Geometry check sheet. Reference: drawing and pictorial views, mm from the part's lowest x, y, z. Round coordinates to 2 decimals unless told otherwise and drop trailing zeros. Order: outer loops, then holes, each group sorted by start corner. A loop starts at its lowest first (then second) coordinate and runs counter-clockwise, first axis right, second up.
(1) Release check for a two-part mould opening along X. For the marked faces 1, 2 and 3 record: +X half, -X half, draft (parallel to the pull), parting line (faces both ways), or undercut.
(2) Sectioned sample at D-D (x = 32.5). Record the boundary of the cut face in (y, z).
(3) Sectioned sample at C-C (z = 5). Record the boundary of the cut face in (x, y).
(4) Go/stop test with flat-tipped pins: pin 1 (2 mm diameter, centred on x = 28, y = 19.5, fed in from -Z); pin 2 (2 mm diameter, centred on x = 19.5, y = 27, fed in from +Z); pin 3 (0.7 mm diameter, centred on x = 12.5, z = 2.5, fed in from +Y); pin 4 (1.1 mm diameter, centred on y = 15, z = 2.5, fed in from -X). Record where each tip stops, or that it passes through.
(5) Sectioned sample at B-B (y = 33). Record the boundary of the cut face in (x, z).
(6) Material ranges on line 1 along X through (y, z) = (35, 2.75); line 2 along Y through (x, z) = (12.5, 1.75); line 3 along X through (y, z) = (24.5, 9), recorded low to high.
(7) Sectioned sample at A-A (x = 6.5). Record the boundary of the cut face in (y, z).
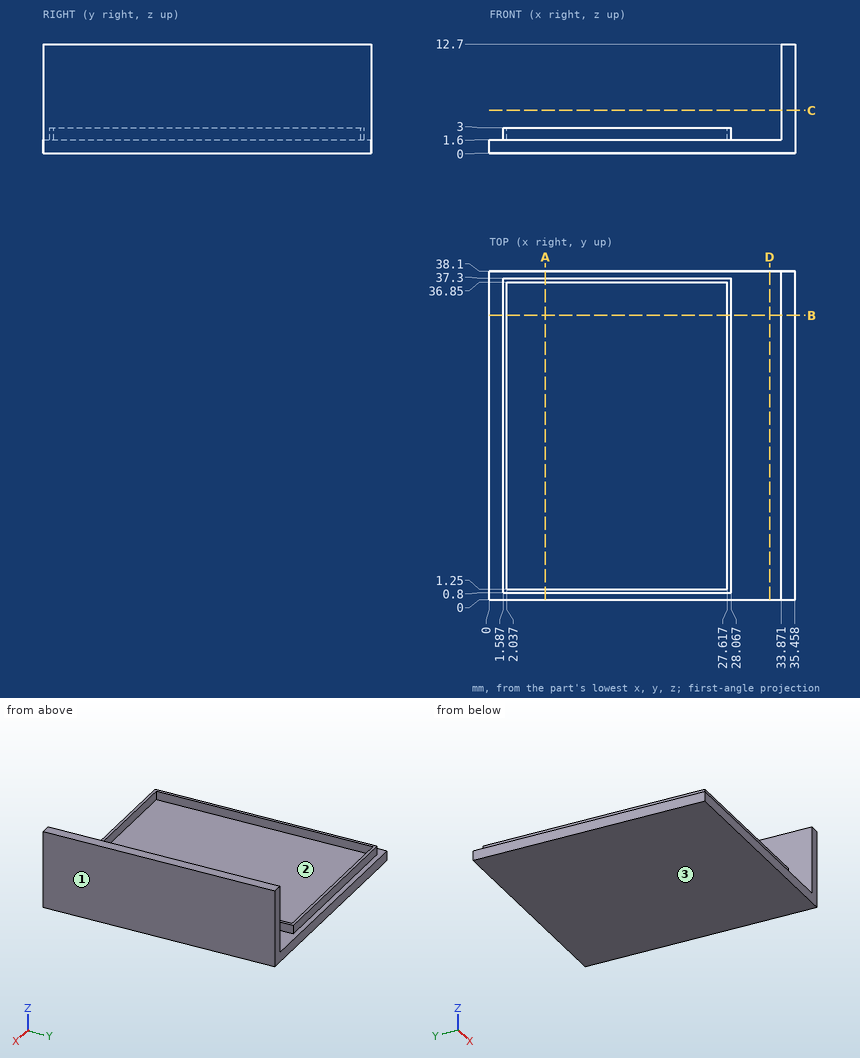
Answer below:
1. face 1: +X half
1. face 2: undercut
1. face 3: draft
2. outline: (0, 0) - (38.1, 0) - (38.1, 1.6) - (0, 1.6) - close
3. outline: (33.87, 0) - (35.46, 0) - (35.46, 38.1) - (33.87, 38.1) - close
4. pin 1: stops at z = 0
4. pin 2: stops at z = 1.6
4. pin 3: stops at y = 37.3
4. pin 4: stops at x = 1.59
5. outline: (0, 0) - (35.46, 0) - (35.46, 12.7) - (33.87, 12.7) - (33.87, 1.6) - (28.07, 1.6) - (28.07, 3) - (27.62, 3) - (27.62, 1.6) - (2.04, 1.6) - (2.04, 3) - (1.59, 3) - (1.59, 1.6) - (0, 1.6) - close
6. line 1: x = 1.59 to 2.04, 27.62 to 28.07, 33.87 to 35.46
6. line 2: y = 0.8 to 1.25, 36.85 to 37.3
6. line 3: x = 33.87 to 35.46
7. outline: (0, 0) - (38.1, 0) - (38.1, 1.6) - (37.3, 1.6) - (37.3, 3) - (36.85, 3) - (36.85, 1.6) - (1.25, 1.6) - (1.25, 3) - (0.8, 3) - (0.8, 1.6) - (0, 1.6) - close
